from build123d import *

# Parameters (mm, degrees)
SKETCH1_W           = 45
SKETCH1_H           = 25
BOSS_EXTRUDE1_DEPTH = 70
SKETCH2_R           = 6
CUT_EXTRUDE1_DEPTH  = 70
SKETCH3_R           = 10
CUT_EXTRUDE2_DEPTH  = 2
SKETCH4_R           = 10
CUT_EXTRUDE3_DEPTH  = 2
SKETCH5_R           = 2.5
CUT_EXTRUDE4_DEPTH  = 15
SKETCH6_R           = 2.5
CUT_EXTRUDE5_DEPTH  = 15
SKETCH7_R           = 2.5
CUT_EXTRUDE6_DEPTH  = 36
SKETCH8_R           = 2.5
CUT_EXTRUDE7_DEPTH  = 38


with BuildPart() as part:
    # Sketch1 → Boss-Extrude1 (new body)
    with BuildSketch(Plane(origin=(0, 0, 0), x_dir=(1, 0, 0), z_dir=(0, 1, 0))):
        Rectangle(SKETCH1_W, SKETCH1_H)
    extrude(amount=BOSS_EXTRUDE1_DEPTH)

    # Sketch2 → Cut-Extrude1 (cut)
    with BuildSketch(Plane(origin=(22.5, 0, 0), x_dir=(0, 0, -1), z_dir=(1, 0, 0))):
        with Locations((0, 52.5)):
            Circle(SKETCH2_R)
        with Locations((0, 17.5)):
            Circle(SKETCH2_R)
    extrude(amount=-CUT_EXTRUDE1_DEPTH, mode=Mode.SUBTRACT)

    # Sketch3 → Cut-Extrude2 (cut)
    with BuildSketch(Plane(origin=(22.5, 0, 0), x_dir=(0, 0, -1), z_dir=(1, 0, 0))):
        with Locations((0, 17.5)):
            Circle(SKETCH3_R)
        with Locations((0, 52.5)):
            Circle(SKETCH3_R)
    extrude(amount=-CUT_EXTRUDE2_DEPTH, mode=Mode.SUBTRACT)

    # Sketch4 → Cut-Extrude3 (cut)
    with BuildSketch(Plane.ZY.offset(22.5)):
        with Locations((0, 52.5)):
            Circle(SKETCH4_R)
        with Locations((0, 17.5)):
            Circle(SKETCH4_R)
    extrude(amount=-CUT_EXTRUDE3_DEPTH, mode=Mode.SUBTRACT)

    # Sketch5 → Cut-Extrude4 (cut)
    with BuildSketch(Plane(origin=(22.5, 0, 0), x_dir=(0, 0, -1), z_dir=(1, 0, 0))):
        with Locations((7.5, 6)):
            Circle(SKETCH5_R)
        with Locations((-7.5, 6)):
            Circle(SKETCH5_R)
        with Locations((7.5, 64)):
            Circle(SKETCH5_R)
        with Locations((-7.5, 64)):
            Circle(SKETCH5_R)
    extrude(amount=-CUT_EXTRUDE4_DEPTH, mode=Mode.SUBTRACT)

    # Sketch6 → Cut-Extrude5 (cut)
    with BuildSketch(Plane(origin=(22.5, 0, 0), x_dir=(0, 0, -1), z_dir=(1, 0, 0))):
        with Locations((0, 35)):
            Circle(SKETCH6_R)
    extrude(amount=-CUT_EXTRUDE5_DEPTH, mode=Mode.SUBTRACT)

    # Sketch7 → Cut-Extrude6 (cut)
    with BuildSketch(Plane.XY.offset(12.5)):
        with Locations((-15.5, 52.5)):
            Circle(SKETCH7_R)
        with Locations((-15.5, 17.5)):
            Circle(SKETCH7_R)
    extrude(amount=-CUT_EXTRUDE6_DEPTH, mode=Mode.SUBTRACT)

    # Sketch8 → Cut-Extrude7 (cut)
    with BuildSketch(Plane.XY.offset(12.5)):
        with Locations((-15.5, 64)):
            Circle(SKETCH8_R)
        with Locations((-15.5, 6)):
            Circle(SKETCH8_R)
    extrude(amount=-CUT_EXTRUDE7_DEPTH, mode=Mode.SUBTRACT)


solid = part.part
Model file for the job. Use its own axes, mm. A direction names the side the tool comes from. Coordinates: 2 decimals unless noted, no trailing zeros. Loops run counter-clockwise (first coordinate to the right, second up) from the corner with the lowest first, then second, coordinate; pieces in that order, holes last. Notation, with made-up numbers: (-17, 82.25) -> (18, 82.25) arc R17 cw to (18, 88.25) -> close; hole circle Ø3 at (28.25, -8.75). An arc over 180 degrees is marked (long way). Use one line per item in the form item = value. Start each with the question number.
(1) Probe probe 1 along Y at (x, z) = (-15.5, -8.5); probe 2 along X at (y, z) = (52.5, -7); probe 3 along Y at (x, z) = (-21.75, 0). List the from-to ranges inside material, lowest first. Write a range as from..to.
(2) Tool access for faces 4 (the flat face through (0, 0, 0)), 5 (the flat face through (7.5, 6, -7)), 6 (the flat face through (-20.5, 46, 0)): list every direction of +Z, -Z, +X, -X, +Y, -Y with a clear straight run to the whole face (end or side of a thin tool).
(3) Cut at A-A on z = 0. Give the number of separate pieces and of enclosed holes in the cut face, and give its area (3 significant figures).
(4) Cut at C-C on x = -19. Give the cut face in (y, z), and give its area (3 significant figures).
(5) Flat gauge pins, fed straight in: pin 1 (4.5 mm diameter, centred on x = -15.5, y = 6, fed in from -Z); pin 2 (10 mm diameter, centred on y = 53.5, z = -1, fed in from -X); pin 3 (4.5 mm diameter, centred on y = 64, z = -7.5, fed in from +X); pin 4 (10 mm diameter, centred on y = 50, z = -1.5, fed in from +X). Where does each tip first touch, or does it go through?
(6) Pull direction Z, two halves, no side cores. Call faces 1 (the flat face through (0, 35, 12.5)), 2 (the cylindrical face through (15.1, 66.48, 7.83)), 3 (the cylindrical face through (-18, 64, 0)): pulls with the +Z half, pulls with the -Z half, needs draft (parallel to the pull), parting line crosses it, or undercut.
(7) Cut at B-B on y = 17.5. Give the cut face in (x, z), and give its area (3 significant figures).
(8) Cut at D-D on y = 64. Give the cut face in (x, z).
Values:
q1.probe_1 = 0..3.5, 8.5..15, 20..50, 55..61.5, 66.5..70
q1.probe_2 = -20.5..-18, -13..20.5
q1.probe_3 = 0..7.5, 27.5..42.5, 62.5..70
q2.face_4 = +Z, -Z, +X, -X, -Y
q2.face_5 = +X
q2.face_6 = -X
q3.separate_pieces = 3
q3.enclosed_holes = 2
q3.area = 1,890 mm2
q4.outline = (0, -12.5) -> (70, -12.5) -> (70, 12.5) -> (0, 12.5) -> close; hole circle Ø12 at (17.5, 0); hole circle Ø12 at (52.5, 0)
q4.area = 1,520 mm2
q5.pin_1 = through
q5.pin_2 = -20.5
q5.pin_3 = 7.5
q5.pin_4 = 20.5
q6.face_1 = pulls with the +Z half
q6.face_2 = undercut
q6.face_3 = needs draft
q7.outline = (-22.5, -12.5) -> (-18, -12.5) -> (-18, -6) -> (-20.5, -6) -> (-20.5, -10) -> (-22.5, -10) -> close; (-22.5, 10) -> (-20.5, 10) -> (-20.5, 6) -> (-18, 6) -> (-18, 12.5) -> (-22.5, 12.5) -> close; (-13, -12.5) -> (22.5, -12.5) -> (22.5, -10) -> (20.5, -10) -> (20.5, -6) -> (-13, -6) -> close; (-13, 6) -> (20.5, 6) -> (20.5, 10) -> (22.5, 10) -> (22.5, 12.5) -> (-13, 12.5) -> close
q7.area = 488 mm2
q8.outline = (-22.5, -12.5) -> (-18, -12.5) -> (-18, 12.5) -> (-22.5, 12.5) -> close; (-13, -12.5) -> (22.5, -12.5) -> (22.5, -10) -> (7.5, -10) -> (7.5, -5) -> (22.5, -5) -> (22.5, 5) -> (7.5, 5) -> (7.5, 10) -> (22.5, 10) -> (22.5, 12.5) -> (-13, 12.5) -> close
